Check sheet for the drawn part. Datum: minimum x, y, z corner. Units: mm. Coordinates: 2 decimals unless noted, no trailing zeros. Write each loop counter-clockwise with the first axis right and the second up, starting at its lowest first coordinate (ties: lowest second). Pieces come first, ordered by that corner, then holes. Notation, with made-up numbers: M 58,85 L 95,85 A31 ccw 95,124 Z; hole C -26,29 d6. An arc over 180 degrees is marked long. Answer as a JSON object with one key per item and string values. Group by question number.
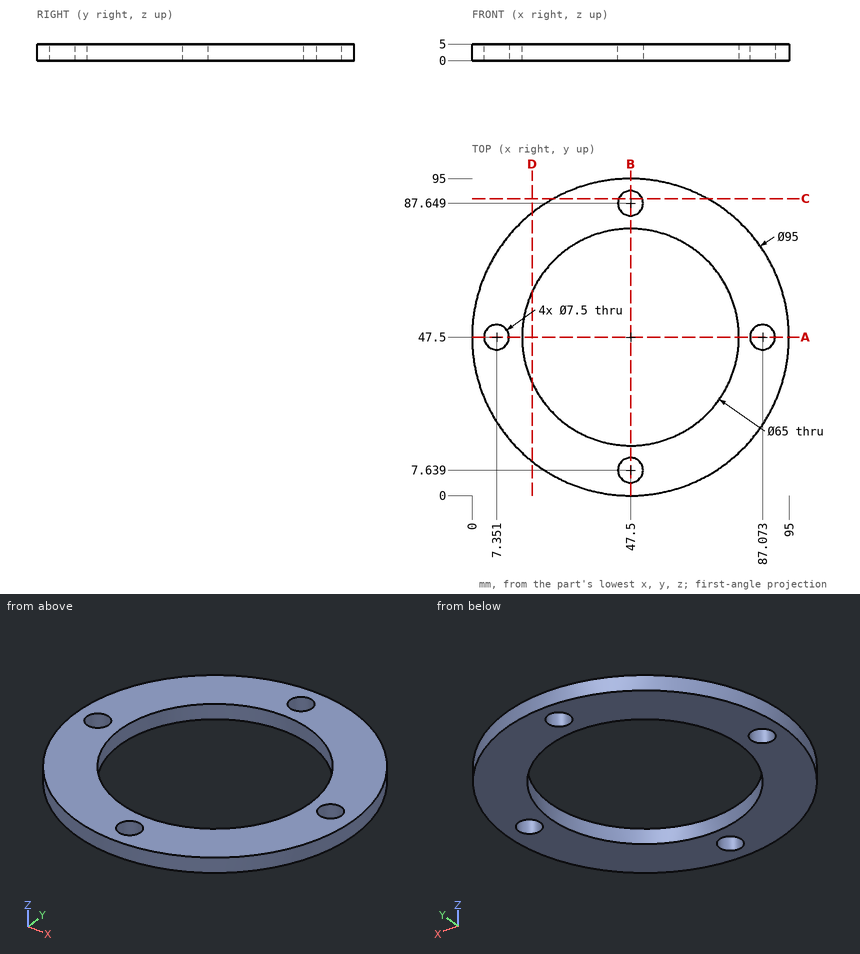
1) Material ranges on probe 1 along Y at (x, z) = (47.5, 3.55); probe 2 along Y at (x, z) = (9.5, 3.6) (1 decimal); probe 3 along X at (y, z) = (86, 3), recorded low to high. Write a range as [from, to].
2) Section check D-D (x = 18). Record the cut outline in (y, z), then the cut area to 3 significant figures.
3) Section check B-B (x = 47.5). Record the cut outline in (y, z), then the cut area to 3 significant figures.
4) Section check C-C (y = 89). Record the cut outline in (x, z), then the cut area to 3 significant figures.
5) Section check A-A (y = 47.5). Record the cut outline in (x, z), then the cut area to 3 significant figures.
6) Go/stop test with flat-tipped pins: pin 1 Ø1.5 at (x, y) = (35.5, 19.5) entering from -Z; pin 2 Ø2 at (x, z) = (45.5, 3) entering from -Y; pin 3 Ø2 at (y, z) = (40.5, 3.5) entering from -X. Record where each tip stops, or that it passes through.
Entries:
{
 "1": {"probe 1": "[0, 3.89], [11.39, 15], [80, 83.9], [91.4, 95]", "probe 2": "[19, 44.4], [50.6, 76]", "probe 3": "[19.68, 44.13], [50.87, 75.32]"},
 "2": {"outline": "M 10.27,0 L 33.86,0 L 33.86,5 L 10.27,5 Z; M 61.14,0 L 84.73,0 L 84.73,5 L 61.14,5 Z", "area": "236 mm^2"},
 "3": {"outline": "M 0,0 L 3.89,0 L 3.89,5 L 0,5 Z; M 11.39,0 L 15,0 L 15,5 L 11.39,5 Z; M 80,0 L 83.9,0 L 83.9,5 L 80,5 Z; M 91.4,0 L 95,0 L 95,5 L 91.4,5 Z", "area": "75.0 mm^2"},
 "4": {"outline": "M 24.39,0 L 44,0 L 44,5 L 24.39,5 Z; M 51,0 L 70.61,0 L 70.61,5 L 51,5 Z", "area": "196 mm^2"},
 "5": {"outline": "M 0,0 L 3.6,0 L 3.6,5 L 0,5 Z; M 11.1,0 L 15,0 L 15,5 L 11.1,5 Z; M 80,0 L 83.32,0 L 83.32,5 L 80,5 Z; M 90.82,0 L 95,0 L 95,5 L 90.82,5 Z", "area": "75.0 mm^2"},
 "6": {"pin 1": "through", "pin 2": "y = 0.01", "pin 3": "x = 0.38"}
}
